Here's how the part is built. I have some questions about the finished solid (model axes, mm). Face numbers are marked on the shaded views. Round coordinates to 2 decimals unless told otherwise and drop trailing zeros. Loops run counter-clockwise (first coordinate to the right, second up) from the corner with the lowest first, then second, coordinate; pieces in that order, holes last. Notation, with made-up numbers: M 29.25,44 L 48.25,44 A27 cw 48.25,73 Z; hole C 34.25,77.5 d10. An arc over 180 degrees is marked long. Use a Markdown table: item, result.
from build123d import *

# Parameters (mm, degrees)
EXTRUDE_1_DEPTH     = 32
SKETCH_2_R          = 2.05
CUT_EXTRUDE_1_DEPTH = 5.1
SKETCH_3_W          = 230
SKETCH_3_H          = 18
CUT_EXTRUDE_2_DEPTH = 8
SKETCH_4_W          = 6
SKETCH_4_H          = 32
SKETCH_4_H_2        = 6
SKETCH_4_H_3        = 43
CUT_EXTRUDE_3_DEPTH = 6
SKETCH_5_R          = 1
CUT_EXTRUDE_4_DEPTH = 38
SKETCH_6_W          = 4
SKETCH_6_H          = 30
CUT_EXTRUDE_5_DEPTH = 335.984621748
CHAMFER_1_SIZE2     = 8
CHAMFER_1_SIZE      = 0.3
CUT_EXTRUDE_6_DEPTH = 258.992463284


with BuildPart() as part:
    # 草图1 → 凸台-拉伸1 (new body)
    with BuildSketch(Plane.XY):
        with BuildLine():
            Line((145.333333333, -27.048611111), (153.333333333, -27.048611111))
            Line((153.333333333, -27.048611111), (153.333333333, 167.951388889))
            ThreePointArc((153.333333333, 167.951388889), (150.404401145, 175.022456701), (143.333333333, 177.951388889))
            Line((143.333333333, 177.951388889), (-126.666666667, 177.951388889))
            ThreePointArc((-126.666666667, 177.951388889), (-133.737734479, 175.022456701), (-136.666666667, 167.951388889))
            Line((-136.666666667, 167.951388889), (-136.666666667, -27.048611111))
            Line((-136.666666667, -27.048611111), (-128.666666667, -27.048611111))
            Line((-128.666666667, -27.048611111), (-128.666666667, 159.951388889))
            ThreePointArc((-128.666666667, 159.951388889), (-125.737734479, 167.022456701), (-118.666666667, 169.951388889))
            Line((-118.666666667, 169.951388889), (135.333333333, 169.951388889))
            ThreePointArc((135.333333333, 169.951388889), (142.404401145, 167.022456701), (145.333333333, 159.951388889))
            Line((145.333333333, 159.951388889), (145.333333333, -27.048611111))
        make_face()
    extrude(amount=EXTRUDE_1_DEPTH)

    # 草图2 → 切除-拉伸1 (cut)
    with BuildSketch(Plane(origin=(0, 0, 0), x_dir=(-1, 0, 0), z_dir=(0, 0, -1))):
        with Locations((132.666666667, 127.951388889)):
            Circle(SKETCH_2_R)
        with Locations((132.666666667, 24.951388889)):
            Circle(SKETCH_2_R)
        with Locations((-149.333333333, 127.951388889)):
            Circle(SKETCH_2_R)
        with Locations((-149.333333333, 24.951388889)):
            Circle(SKETCH_2_R)
        with Locations((-135.333333333, 173.951388889)):
            Circle(SKETCH_2_R)
        with Locations((-8.333333333, 173.951388889)):
            Circle(SKETCH_2_R)
        with Locations((118.666666667, 173.951388889)):
            Circle(SKETCH_2_R)
    extrude(amount=-CUT_EXTRUDE_1_DEPTH, mode=Mode.SUBTRACT)

    # 草图3 → 切除-拉伸2 (cut)
    with BuildSketch(Plane(origin=(0, 177.951388889, 0), x_dir=(1, 0, 0), z_dir=(0, 1, 0))):
        with Locations((8.333333333, -9)):
            Rectangle(SKETCH_3_W, SKETCH_3_H)
    extrude(amount=-CUT_EXTRUDE_2_DEPTH, mode=Mode.SUBTRACT)

    # 草图4 → 切除-拉伸3 (cut)
    with BuildSketch(Plane.ZY.offset(136.666666667)):
        with Locations((29, 72.951388889)):
            Rectangle(SKETCH_4_W, SKETCH_4_H)
        with Locations((29, 94.951388889)):
            Rectangle(SKETCH_4_W, SKETCH_4_H_2)
        with Locations((29, 32.451388889)):
            Rectangle(SKETCH_4_W, SKETCH_4_H_3)
    extrude(amount=-CUT_EXTRUDE_3_DEPTH, mode=Mode.SUBTRACT)

    # 草图5 → 切除-拉伸4 (cut)
    with BuildSketch(Plane.XZ.offset(-53.951388889)):
        with Locations(Location((-134.666666667, 29, 0), (0, 0, 270))):
            Circle(SKETCH_5_R)
    extrude(amount=-CUT_EXTRUDE_4_DEPTH, mode=Mode.SUBTRACT)

    # 草图6 → 切除-拉伸5 (cut, through all)
    with BuildSketch(Plane.ZY.offset(-145.333333333)):
        with Locations((16.078720605, 93.951388889)):
            Rectangle(SKETCH_6_W, SKETCH_6_H)
    extrude(amount=-CUT_EXTRUDE_5_DEPTH, mode=Mode.SUBTRACT)

    # 倒角1
    chamfer_1_edges = [part.edges().sort_by_distance(p)[0] for p in [
        (145.333333333, 93.951388889, 18.078720605),
    ]]
    chamfer_1_side = [part.faces().sort_by_distance(p)[0] for p in [
        (145.333333333, 93.951388889, 18.084720605),
    ]]
    chamfer(chamfer_1_edges, length=CHAMFER_1_SIZE - 0.0001, length2=CHAMFER_1_SIZE2 - 0.0001, reference=chamfer_1_side[0])  # a hair under: the kernel refuses the full size

    # 草图7 → 切除-拉伸6 (cut, through all)
    with BuildSketch(Plane(origin=(0, 177.951388889, 0), x_dir=(1, 0, 0), z_dir=(0, 1, 0))):
        with BuildLine():
            Line((-136.666666667, -28.7), (-136.666666667, -32))
            Line((-136.666666667, -32), (-133.366666667, -32))
            ThreePointArc((-133.366666667, -32), (-135.700119045, -31.033452378), (-136.666666667, -28.7))
        make_face()
    extrude(amount=-CUT_EXTRUDE_6_DEPTH, mode=Mode.SUBTRACT)


solid = part.part
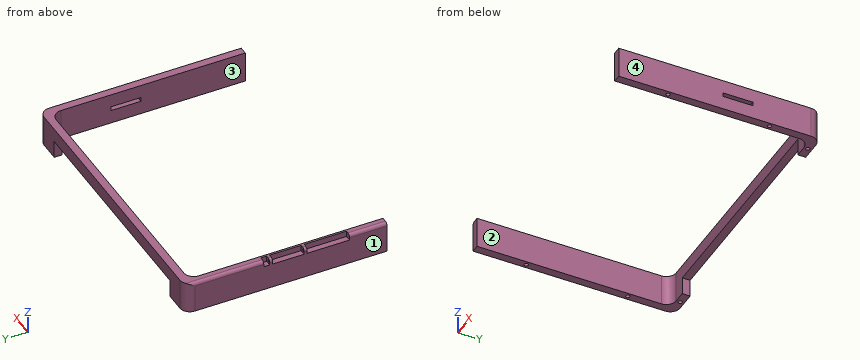
1. We'd pull the mould along X, two halves only. Please class the marked faces 1, 2, 3 and 4: +X half, -X half, draft (parallel to the pull), parting line (faces both ways), or undercut.
Answer sheet:
| item | result |
|---|---|
| face 1 | -X half |
| face 2 | undercut |
| face 3 | undercut |
| face 4 | +X half |
2. Imagine slicing it at B-B, the plane y = 34. Write out the boundary of the cut face in (x, z).
Answer sheet:
| item | result |
|---|---|
| outline | M -136.67,0 L -128.67,0 L -128.67,32 L -130.67,32 L -130.67,26 L -136.67,26 Z; M 145.33,0 L 153.33,0 L 153.33,32 L 145.33,32 Z |
3. Imagine slicing it at A-A, the plane y = 3. Write out the boundary of the cut face in (x, z).
Answer sheet:
| item | result |
|---|---|
| outline | M -136.67,0 L -128.67,0 L -128.67,32 L -133.37,32 A3.3 ccw -136.67,28.7 Z; M 145.33,0 L 153.33,0 L 153.33,32 L 145.33,32 Z |
4. For pin 1 Ø3 at (x, y) = (-133, 80.5) entering from +Z; pin 2 Ø3.5 at (x, y) = (149.33, 24.95) entering from -Z; pin 3 Ø4.5 at (x, z) = (148.5, 16.5) entering from +Y; pin 4 Ø6 at (x, z) = (-103, 5.5) entering from +Y, each with a flat end and sliding along its axis, tell me the tip position at first contact or that it passes through.
Answer sheet:
| item | result |
|---|---|
| pin 1 | z = 26 |
| pin 2 | z = 5.1 |
| pin 3 | y = 177.52 |
| pin 4 | through |
5. I need wall thicknesses on probe 1 along X at (y, z) = (136.5, 4); probe 2 along X at (y, z) = (37.5, 26.5); probe 3 along Y at (x, z) = (-43, 29). Which ranges of each line are inside material? Lowest first, please. Write a range as from..to.
Answer sheet:
| item | result |
|---|---|
| probe 1 | -136.67..-128.67, 145.33..153.33 |
| probe 2 | -130.67..-128.67, 145.33..153.33 |
| probe 3 | 169.95..177.95 |
6. Imagine slicing it at C-C, the plane x = 116. Write out the boundary of the cut face in (y, z).
Answer sheet:
| item | result |
|---|---|
| outline | M 169.95,18 L 177.95,18 L 177.95,32 L 169.95,32 Z |
